Input: part model. Units: mm. Frame: model coordinates. Face numbers are marked on the shaded views. Round coordinates to 2 decimals unless told otherwise and drop trailing zeros. Order: outer loops, then holes, each group sorted by start corner. A loop starts at its lowest first (then second) coordinate and runs counter-clockwise, first axis right, second up. Notation, with made-up numbers: (61.5, 68.5) -> (101.5, 68.5) arc R18 ccw to (101.5, 102.5) -> close; hole circle Ø7 at (-22.75, -7). An arc over 180 degrees is marked (long way). Use a Markdown table: item, result.
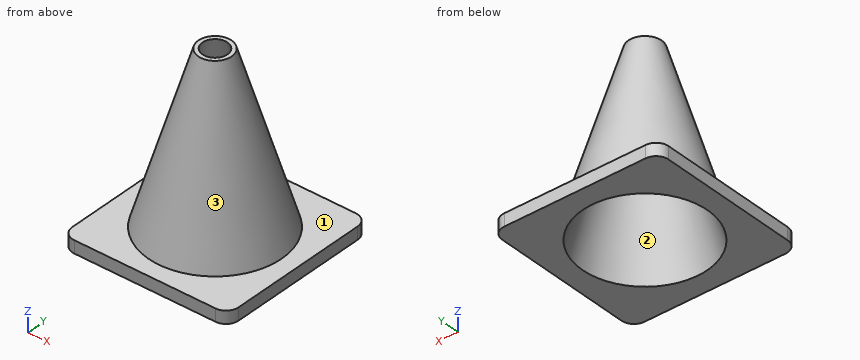
from build123d import *

# Parameters (mm, degrees)
BOX_W     = 40
BOX_H     = 40
BOX_DEPTH = 3
FILLET_R  = 3


with BuildPart() as cono_interior:
    # Cone002 → Cone002 (revolve)
    with BuildSketch(Plane(origin=(20, 20, 0), x_dir=(1, 0, 0), z_dir=(0, -1, 0))):
        Polygon((0, 0), (15, 0), (3, 43), (0, 43), align=None)
    revolve(axis=Axis((20, 20, 0), (0, 0, 1)))


with BuildPart() as cono_ext:
    # Cone → Cone (revolve)
    with BuildSketch(Plane(origin=(20, 20, 3), x_dir=(1, 0, 0), z_dir=(0, -1, 0))):
        Polygon((0, 0), (16, 0), (4, 40), (0, 40), align=None)
    revolve(axis=Axis((20, 20, 3), (0, 0, 1)))


with BuildPart() as obj1:
    # Box → Box (new body)
    with BuildSketch(Plane.XY):
        with Locations((20, 20)):
            Rectangle(BOX_W, BOX_H)
    extrude(amount=BOX_DEPTH)

    # Fusion: union Cono_ext
    add(cono_ext.part)

    # Cut: cut Cono_interior
    add(cono_interior.part, mode=Mode.SUBTRACT)

    # Fillet
    fillet_edges = [obj1.edges().sort_by_distance(p)[0] for p in [
        (0, 0, 1.5),
        (0, 40, 1.5),
        (40, 0, 1.5),
        (40, 40, 1.5),
    ]]
    fillet(fillet_edges, radius=FILLET_R)


solid = obj1.part
1) Pull-direction query (X, two-part tool) for the marked faces 1, 2 and 3; classes: +X half, -X half, draft (parallel to the pull), parting line (faces both ways), or undercut.
Results found:
| item | result |
|---|---|
| face 1 | draft |
| face 2 | undercut |
| face 3 | parting line |
2) Line query: L1, parallel to Z at x = 5.5, y = 34; L2, parallel to X at y = 10, z = 13; L3, parallel to X at y = 21, z = 34. Output: solid intervals per line, ascending. Write a range as [from, to].
Results found:
| item | result |
|---|---|
| L1 | z = [0, 3] |
| L2 | x = [11.69, 14.58], [25.42, 28.31] |
| L3 | x = [13.38, 14.58], [25.42, 26.62] |
3) Pin query (flat end, axial travel): pin 1 Ø1 at (x, z) = (14.5, 9.5) entering from +Y; pin 2 Ø10 at (y, z) = (10, 9) entering from +X; pin 3 Ø1.5 at (y, z) = (14, 20) entering from -X. Return the tip coordinate at first contact, or that it passes through.
Results found:
| item | result |
|---|---|
| pin 1 | stops at y = 33.19 |
| pin 2 | stops at x = 33.86 |
| pin 3 | stops at x = 10.37 |
4) Cut plane D-D on z = 35. Return loops of the section in (x, y), and give its area (3 significant figures).
Results found:
| item | result |
|---|---|
| outline | circle Ø12.8 at (20, 20); hole circle Ø10.47 at (20, 20) |
| area | 42.7 mm² |
5) Cut plane A-A on x = 20. Return loops of the section in (y, z).
Results found:
| item | result |
|---|---|
| outline | (0, 0) -> (5, 0) -> (17, 43) -> (16, 43) -> (4, 3) -> (0, 3) -> close; (23, 43) -> (35, 0) -> (40, 0) -> (40, 3) -> (36, 3) -> (24, 43) -> close |
6) Cut plane C-C on z = 12. Return loops of the section in (x, y).
Results found:
| item | result |
|---|---|
| outline | circle Ø26.6 at (20, 20); hole circle Ø23.3 at (20, 20) |
